Geometry: final body of the model. Coordinates: model frame, mm. Give positions to 0.01 mm unless a question says otherwise; leave off trailing zeros. Loops run counter-clockwise (first coordinate to the right, second up) from the corner with the lowest first, then second, coordinate; pieces in that order, holes last.
from build123d import *

# Parameters (mm, degrees)
F0_R     = 12.7
F0_R_2   = 44.45
F1_DEPTH = 6.35


with BuildPart() as f1:
    # F0 (on Top) → F1 (new body)
    with BuildSketch(Plane.XY):
        with BuildLine():
            ThreePointArc((-78.214847, -34.462572), (-61.091134, -35.359671), (-46.095031, -43.674914))
            ThreePointArc((-46.095031, -43.674914), (-44.727285, -44.969636), (-43.42519, -46.330367))
            ThreePointArc((-43.42519, -46.330367), (4.393779, -63.347807), (49.405516, -39.891665))
            ThreePointArc((49.405516, -39.891665), (61.271133, -33.539825), (74.60493, -31.709908))
            ThreePointArc((74.60493, -31.709908), (107.949523, -0.174093), (74.952768, 31.725493))
            ThreePointArc((74.952768, 31.725493), (59.918318, 34.310355), (47.103013, 42.585869))
            ThreePointArc((47.103013, 42.585869), (46.088419, 43.617938), (45.113755, 44.687796))
            ThreePointArc((45.113755, 44.687796), (-7.094296, 63.102464), (-53.910206, 33.555024))
            ThreePointArc((-53.910206, 33.555024), (-64.305996, 29.254689), (-75.504467, 28.177844))
            ThreePointArc((-75.504467, 28.177844), (-113.602257, -1.552553), (-78.214847, -34.462572))
        make_face()
        with Locations((-81.881937, -2.925055)):
            Circle(F0_R, mode=Mode.SUBTRACT)
        Circle(F0_R_2, mode=Mode.SUBTRACT)
        with BuildLine():
            ThreePointArc((88.9, 0), (76.2, -12.7), (63.5, 0))
            ThreePointArc((63.5, 0), (76.2, 12.7), (88.9, 0))
        make_face(mode=Mode.SUBTRACT)
    extrude(amount=F1_DEPTH)


solid = f1.part
Item 1: Section query A-A on x = 0. Return loops of the section in (y, z), plus the area to 3 significant figures.
Values follow:
outline: (-63.5, 0) - (-44.45, 0) - (-44.45, 6.35) - (-63.5, 6.35) - close; (44.45, 0) - (63.5, 0) - (63.5, 6.35) - (44.45, 6.35) - close
area: 242 mm2
Item 2: Draft query along X for faces 1 (the face through (3.664, -63.394, 3.131)), 2 (the face through (45, 1, 6.35)), 3 (the face through (42.397, 13.352, 3.131)). Return one class per face: +X half, -X half, draft (parallel to the pull), parting line (faces both ways), or undercut.
Values follow:
face 1: parting line
face 2: draft
face 3: undercut
Item 3: Section query C-C on y = 37.5. Return loops of the section in (x, z), plus the area to 3 significant figures.
Values follow:
outline: (-51.24, 0) - (-23.87, 0) - (-23.87, 6.35) - (-51.24, 6.35) - close; (23.87, 0) - (53.56, 0) - (53.56, 6.35) - (23.87, 6.35) - close
area: 362 mm2
Item 4: Ray query, probe 1 along Y at (x, z) = (76.2, 2.25); probe 2 along X at (y, z) = (-2.5, 0.5); probe 3 along X at (y, z) = (15.5, 4.75). Return the intervals inside material, ascending.
Values follow:
probe 1: y = -31.75 to -12.7, 12.7 to 31.75
probe 2: x = -113.63 to -94.57, -69.19 to -44.38, 44.38 to 63.75, 88.65 to 107.85
probe 3: x = -107.74 to -41.66, 41.66 to 103.91
Item 5: Pin query (flat end, axial travel): pin 1 (3 mm diameter, centred on y = 49, z = 5, fed in from -X); pin 2 (23 mm diameter, centred on x = -81.88, y = -2.93, fed in from -Z); pin 3 (1 mm diameter, centred on y = 42, z = 4, fed in from +X); pin 4 (3 mm diameter, centred on x = -14, y = 45, fed in from -Z). Return the tip coordinate at first contact, or that it passes through.
Values follow:
pin 1: stops at x = -42.14
pin 2: passes through
pin 3: stops at x = 48.26
pin 4: stops at z = 0
Item 6: Section query B-B on z = 1.5. Return loops of the section in (x, y).
Values follow:
outline: (-78.21, -34.46) arc R38.1 cw to (-46.1, -43.67) arc R38.1 cw to (-43.43, -46.33) arc R63.5 ccw to (49.41, -39.89) arc R38.1 cw to (74.6, -31.71) arc R31.75 ccw (long way) to (74.95, 31.73) arc R38.1 cw to (47.1, 42.59) arc R38.1 cw to (45.11, 44.69) arc R63.5 ccw to (-53.91, 33.56) arc R38.1 cw to (-75.5, 28.18) arc R31.75 ccw (long way) to start; hole circle Ø25.4 at (-81.88, -2.93); hole circle Ø88.9 at (0, 0); hole circle Ø25.4 at (76.2, 0)
Item 7: Section query D-D on y = 0. Return loops of the section in (x, z), plus the area to 3 significant figures.
Values follow:
outline: (-113.5, 0) - (-94.24, 0) - (-94.24, 6.35) - (-113.5, 6.35) - close; (-69.52, 0) - (-44.45, 0) - (-44.45, 6.35) - (-69.52, 6.35) - close; (44.45, 0) - (63.5, 0) - (63.5, 6.35) - (44.45, 6.35) - close; (88.9, 0) - (107.95, 0) - (107.95, 6.35) - (88.9, 6.35) - close
area: 523 mm2
